The model under review builds one solid part; all positions refer to its coordinate system, in mm. Round coordinates to 2 decimals unless told otherwise and drop trailing zeros. Write each loop counter-clockwise with the first axis right and the second up, starting at its lowest first coordinate (ties: lowest second). Pieces come first, ordered by that corner, then holes.
Item 1: Add section A-A (z = -4.05). Give the boundary of the cut face in (x, y).
Item 2: Clearance check with flat-ended pins moving along their axes: pin 1 Ø2 at (y, z) = (2, -4.5) entering from +X; pin 2 Ø3 at (x, z) = (18.5, -4.5) entering from -Y. State where each tip first meets the part, or that it passes through.
Item 3: Add section B-B (y = 0.85). State how many separate pieces and enclosed holes the cut face has, plus the area to 3 significant figures.
Item 4: Draft analysis for pull direction Z (two halves, no side actions). For faces 1 (the face through (1.45, 1.97, -2.19)), 2 (the face through (0.86, 2.03, -5.1)), 3 (the face through (19, 4, -3)), state which applies: +Z half, -Z half, draft (parallel to the pull), parting line (faces both ways), or undercut.
Item 5: Add section C-C (z = -2). Give the boundary of the cut face in (x, y).
Item 6: To check wall thickness, follow L1, parallel to X at y = 2.95, z = -3; L2, parallel to X at y = 1.95, z = -3.95; L3, parallel to Z at x = 36, y = 0.95. State the ranges of each line that lie inside material, in increasing order.
Item 7: Add section D-D (z = -0.35). Give the boundary of the cut face in (x, y).
```python
from build123d import *

# Parameters (mm, degrees)
CROQUIS1_W              = 38
CROQUIS1_H              = 6
CROQUIS1_R              = 1.75
SALIENTE_EXTRUIR1_DEPTH = 4
REDONDEO1_R             = 3


with BuildPart() as part:
    # Croquis1 → Saliente-Extruir1 (new body)
    with BuildSketch(Plane(origin=(0, 0, 0), x_dir=(1, 0, 0), z_dir=(0, 1, 0))):
        with Locations((19, 3)):
            Rectangle(CROQUIS1_W, CROQUIS1_H)
        with Locations(Location((3, 3, 0), (0, 0, 270))):
            Circle(CROQUIS1_R, mode=Mode.SUBTRACT)
        with Locations(Location((35, 3, 0), (0, 0, 270))):
            Circle(CROQUIS1_R, mode=Mode.SUBTRACT)
    extrude(amount=SALIENTE_EXTRUIR1_DEPTH)

    # Redondeo1
    redondeo1_edges = [part.edges().sort_by_distance(p)[0] for p in [
        (38, 2, -6),
        (38, 2, 0),
        (0, 2, -6),
        (0, 2, 0),
    ]]
    fillet(redondeo1_edges, radius=REDONDEO1_R - 0.0001)  # a hair under: the kernel refuses the full size


solid = part.part
```
Numbers:
1. outline: (0.19, 0) - (1.6, 0) - (1.6, 4) - (0.19, 4) - close; (4.4, 0) - (33.6, 0) - (33.6, 4) - (4.4, 4) - close; (36.4, 0) - (37.81, 0) - (37.81, 4) - (36.4, 4) - close
2. pin 1: stops at x = 37.96
2. pin 2: stops at y = 0
3. separate pieces: 1
3. enclosed holes: 2
3. area: 201 mm2
4. face 1: undercut
4. face 2: -Z half
4. face 3: draft
5. outline: (0.17, 0) - (1.56, 0) - (1.56, 4) - (0.17, 4) - close; (4.44, 0) - (33.56, 0) - (33.56, 4) - (4.44, 4) - close; (36.44, 0) - (37.83, 0) - (37.83, 4) - (36.44, 4) - close
6. L1: x = 0 to 1.25, 4.75 to 33.25, 36.75 to 38
6. L2: x = 0.15 to 1.53, 4.47 to 33.53, 36.47 to 37.85
6. L3: z = -5.83 to -4.44, -1.56 to -0.17
7. outline: (1.59, 0) - (36.41, 0) - (36.41, 4) - (1.59, 4) - close
